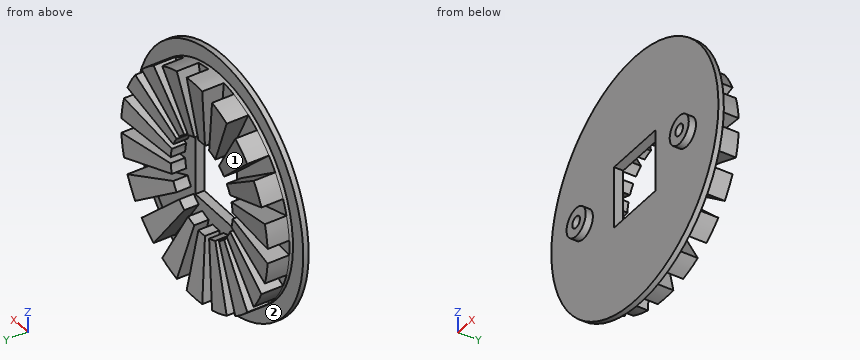
```python
from build123d import *

# Parameters (mm, degrees)
SKETCH2_R           = 15.35
BOSS_EXTRUDE3_DEPTH = 1.25
SKETCH5_W           = 8.7
SKETCH5_H           = 8.7
CUT_EXTRUDE3_DEPTH  = 1.25
BOSS_EXTRUDE4_DEPTH = 4.25
SKETCH1_R           = 17.5
SKETCH1_R_2         = 15.35
BOSS_EXTRUDE5_DEPTH = 0.75
SKETCH8_R           = 2
SKETCH8_R_2         = 0.8
BOSS_EXTRUDE6_DEPTH = 1


with BuildPart() as part:
    # Sketch2 → Boss-Extrude3 (new body)
    with BuildSketch(Plane(origin=(0, 0, 0), x_dir=(1, 0, 0), z_dir=(0, 1, 0))):
        with Locations(Location((0, 0, 0), (0, 0, 270))):
            Circle(SKETCH2_R)
    extrude(amount=BOSS_EXTRUDE3_DEPTH)

    # Sketch5 → Cut-Extrude3 (cut)
    with BuildSketch(Plane(origin=(0, 0, 0), x_dir=(-1, 0, 0), z_dir=(0, 1, 0))):
        Rectangle(SKETCH5_W, SKETCH5_H)
    extrude(amount=CUT_EXTRUDE3_DEPTH, mode=Mode.SUBTRACT)

    # Sketch3 → Boss-Extrude4 (add)
    with BuildSketch(Plane(origin=(0, 0, 0), x_dir=(1, 0, 0), z_dir=(0, 1, 0))):
        with BuildLine():
            Line((-1.631153495, 15.263087442), (-0.690716464, 6.463196637))
            ThreePointArc((-0.690716464, 6.463196637), (0, 6.5), (0.690716464, 6.463196637))
            Line((0.690716464, 6.463196637), (1.631153495, 15.263087442))
            ThreePointArc((1.631153495, 15.263087442), (0, 15.35), (-1.631153495, 15.263087442))
        make_face()
        with BuildLine():
            Line((3.687500452, 14.900497992), (1.561482276, 6.30965713))
            ThreePointArc((1.561482276, 6.30965713), (2.223130932, 6.108002035), (2.859604604, 5.837179242))
            Line((2.859604604, 5.837179242), (6.753066257, 13.784723288))
            ThreePointArc((6.753066257, 13.784723288), (5.2500092, 14.424281729), (3.687500452, 14.900497992))
        make_face()
        with BuildLine():
            Line((8.561387423, 12.740688576), (3.625343208, 5.395079853))
            ThreePointArc((3.625343208, 5.395079853), (4.178119463, 4.97928888), (4.683582226, 4.507111884))
            Line((4.683582226, 4.507111884), (11.060459564, 10.643718064))
            ThreePointArc((11.060459564, 10.643718064), (9.866789809, 11.758782202), (8.561387423, 12.740688576))
        make_face()
        with BuildLine():
            Line((12.402644718, 9.044164085), (5.251934245, 3.829776323))
            ThreePointArc((5.251934245, 3.829776323), (5.629165125, 3.25), (5.942650709, 2.633420314))
            Line((5.942650709, 2.633420314), (14.033798213, 6.218923357))
            ThreePointArc((14.033798213, 6.218923357), (13.293489948, 7.675), (12.402644718, 9.044164085))
        make_face()
        with BuildLine():
            Line((14.747960016, 4.256779928), (6.245064502, 1.802545246))
            ThreePointArc((6.245064502, 1.802545246), (6.401250395, 1.128713155), (6.484947812, 0.442099389))
            Line((6.484947812, 0.442099389), (15.31445368, 1.044034712))
            ThreePointArc((15.31445368, 1.044034712), (15.116799009, 2.665499527), (14.747960016, 4.256779928))
        make_face()
        with BuildLine():
            Line((15.31445368, -1.044034712), (6.484947812, -0.442099389))
            ThreePointArc((6.484947812, -0.442099389), (6.401250395, -1.128713155), (6.245064502, -1.802545246))
            Line((6.245064502, -1.802545246), (14.747960016, -4.256779928))
            ThreePointArc((14.747960016, -4.256779928), (15.116799009, -2.665499527), (15.31445368, -1.044034712))
        make_face()
        with BuildLine():
            Line((14.033798213, -6.218923357), (5.942650709, -2.633420314))
            ThreePointArc((5.942650709, -2.633420314), (5.629165125, -3.25), (5.251934245, -3.829776323))
            Line((5.251934245, -3.829776323), (12.402644718, -9.044164085))
            ThreePointArc((12.402644718, -9.044164085), (13.293489948, -7.675), (14.033798213, -6.218923357))
        make_face()
        with BuildLine():
            Line((11.060459564, -10.643718064), (4.683582226, -4.507111884))
            ThreePointArc((4.683582226, -4.507111884), (4.178119463, -4.97928888), (3.625343208, -5.395079853))
            Line((3.625343208, -5.395079853), (8.561387423, -12.740688576))
            ThreePointArc((8.561387423, -12.740688576), (9.866789809, -11.758782202), (11.060459564, -10.643718064))
        make_face()
        with BuildLine():
            Line((6.753066257, -13.784723288), (2.859604604, -5.837179242))
            ThreePointArc((2.859604604, -5.837179242), (2.223130932, -6.108002035), (1.561482276, -6.30965713))
            Line((1.561482276, -6.30965713), (3.687500452, -14.900497992))
            ThreePointArc((3.687500452, -14.900497992), (5.2500092, -14.424281729), (6.753066257, -13.784723288))
        make_face()
        with BuildLine():
            Line((1.631153495, -15.263087442), (0.690716464, -6.463196637))
            ThreePointArc((0.690716464, -6.463196637), (0, -6.5), (-0.690716464, -6.463196637))
            Line((-0.690716464, -6.463196637), (-1.631153495, -15.263087442))
            ThreePointArc((-1.631153495, -15.263087442), (0, -15.35), (1.631153495, -15.263087442))
        make_face()
        with BuildLine():
            Line((-3.687500452, -14.900497992), (-1.561482276, -6.30965713))
            ThreePointArc((-1.561482276, -6.30965713), (-2.223130932, -6.108002035), (-2.859604604, -5.837179242))
            Line((-2.859604604, -5.837179242), (-6.753066257, -13.784723288))
            ThreePointArc((-6.753066257, -13.784723288), (-5.2500092, -14.424281729), (-3.687500452, -14.900497992))
        make_face()
        with BuildLine():
            Line((-8.561387423, -12.740688576), (-3.625343208, -5.395079853))
            ThreePointArc((-3.625343208, -5.395079853), (-4.178119463, -4.97928888), (-4.683582226, -4.507111884))
            Line((-4.683582226, -4.507111884), (-11.060459564, -10.643718064))
            ThreePointArc((-11.060459564, -10.643718064), (-9.866789809, -11.758782202), (-8.561387423, -12.740688576))
        make_face()
        with BuildLine():
            Line((-12.402644718, -9.044164085), (-5.251934245, -3.829776323))
            ThreePointArc((-5.251934245, -3.829776323), (-5.629165125, -3.25), (-5.942650709, -2.633420314))
            Line((-5.942650709, -2.633420314), (-14.033798213, -6.218923357))
            ThreePointArc((-14.033798213, -6.218923357), (-13.293489948, -7.675), (-12.402644718, -9.044164085))
        make_face()
        with BuildLine():
            Line((-14.747960016, -4.256779928), (-6.245064502, -1.802545246))
            ThreePointArc((-6.245064502, -1.802545246), (-6.401250395, -1.128713155), (-6.484947812, -0.442099389))
            Line((-6.484947812, -0.442099389), (-15.31445368, -1.044034712))
            ThreePointArc((-15.31445368, -1.044034712), (-15.116799009, -2.665499527), (-14.747960016, -4.256779928))
        make_face()
        with BuildLine():
            Line((-15.31445368, 1.044034712), (-6.484947812, 0.442099389))
            ThreePointArc((-6.484947812, 0.442099389), (-6.401250395, 1.128713155), (-6.245064502, 1.802545246))
            Line((-6.245064502, 1.802545246), (-14.747960016, 4.256779928))
            ThreePointArc((-14.747960016, 4.256779928), (-15.116799009, 2.665499527), (-15.31445368, 1.044034712))
        make_face()
        with BuildLine():
            Line((-14.033798213, 6.218923357), (-5.942650709, 2.633420314))
            ThreePointArc((-5.942650709, 2.633420314), (-5.629165125, 3.25), (-5.251934245, 3.829776323))
            Line((-5.251934245, 3.829776323), (-12.402644718, 9.044164085))
            ThreePointArc((-12.402644718, 9.044164085), (-13.293489948, 7.675), (-14.033798213, 6.218923357))
        make_face()
        with BuildLine():
            Line((-11.060459564, 10.643718064), (-4.683582226, 4.507111884))
            ThreePointArc((-4.683582226, 4.507111884), (-4.178119463, 4.97928888), (-3.625343208, 5.395079853))
            Line((-3.625343208, 5.395079853), (-8.561387423, 12.740688576))
            ThreePointArc((-8.561387423, 12.740688576), (-9.866789809, 11.758782202), (-11.060459564, 10.643718064))
        make_face()
        with BuildLine():
            Line((-6.753066257, 13.784723288), (-2.859604604, 5.837179242))
            ThreePointArc((-2.859604604, 5.837179242), (-2.223130932, 6.108002035), (-1.561482276, 6.30965713))
            Line((-1.561482276, 6.30965713), (-3.687500452, 14.900497992))
            ThreePointArc((-3.687500452, 14.900497992), (-5.2500092, 14.424281729), (-6.753066257, 13.784723288))
        make_face()
    extrude(amount=BOSS_EXTRUDE4_DEPTH)

    # Sketch7 → Cut-Revolve1 (revolve, cut)
    with BuildSketch(Plane.XY, mode=Mode.PRIVATE) as cut_revolve1_sk:
        Polygon((6.5, 3.25), (15.31445368, 4.25), (6.5, 4.25), align=None)
    revolve(cut_revolve1_sk.sketch.rotate(Axis((0, 3.25, 0), (0, 1, 0)), 83.9), axis=Axis((0, 3.25, 0), (0, 1, 0)), mode=Mode.SUBTRACT)

    # Sketch1 → Boss-Extrude5 (add)
    with BuildSketch(Plane(origin=(0, 0, 0), x_dir=(1, 0, 0), z_dir=(0, 1, 0))):
        with Locations(Location((0, 0, 0), (0, 0, 270))):
            Circle(SKETCH1_R)
        with Locations(Location((0, 0, 0), (0, 0, 83.9))):
            Circle(SKETCH1_R_2, mode=Mode.SUBTRACT)
    extrude(amount=BOSS_EXTRUDE5_DEPTH)

    # Sketch8 → Boss-Extrude6 (add)
    # profile 1 of 2: a face of its own
    with BuildSketch(Plane(origin=(0, 0, 0), x_dir=(1, 0, 0), z_dir=(0, 1, 0))):
        with Locations(Location((-10.8, 0, 0), (0, 0, 270))):
            Circle(SKETCH8_R)
        with Locations(Location((-10.8, 0, 0), (0, 0, 270))):
            Circle(SKETCH8_R_2, mode=Mode.SUBTRACT)
    # profile 2 of 2: a face of its own
    with BuildSketch(Plane(origin=(0, 0, 0), x_dir=(1, 0, 0), z_dir=(0, 1, 0))):
        with Locations(Location((10.8, 0, 0), (0, 0, 90))):
            Circle(SKETCH8_R)
        with Locations(Location((10.8, 0, 0), (0, 0, 270))):
            Circle(SKETCH8_R_2, mode=Mode.SUBTRACT)
    extrude(amount=-BOSS_EXTRUDE6_DEPTH)


solid = part.part
```
Could you check a few things on this model? Use its own coordinates, in mm. Face numbers are marked on the shaded views. Round coordinates to 2 decimals unless told otherwise and drop trailing zeros. Loops run counter-clockwise (first coordinate to the right, second up) from the corner with the lowest first, then second, coordinate; pieces in that order, holes last. Notation, with made-up numbers: (-13.5, 50.25) - (42.5, 50.25) arc R26 ccw to (42.5, 83.25) - close; hole circle Ø1 at (-37, -20.5). An arc over 180 degrees is marked (long way). Answer in a Markdown table with one row per item. Add a question column.
(1) If we mould it in two halves opening along X, with no side actions, what happens to the marked faces 1 and 2? For each: pulls with the +X half, pulls with the -X half, needs draft (parallel to the pull), parting line crosses it, or undercut.
(2) If we section it at B-B (y = 2.35): State how many separate pieces and enclosed holes the cut face has, plus the area to 3 significant figures.
(3) I'm going to push flat-ended pins straight in: pin 1 (2 mm diameter, centred on y = 1, z = -11, fed in from -X); pin 2 (1.5 mm diameter, centred on x = -2.5, y = 0.5, fed in from +Z); pin 3 (4 mm diameter, centred on x = -5, z = -8.5, fed in from -Y); pin 4 (1.8 mm diameter, centred on x = 10.8, z = 0, fed in from -Y). Where does each tip first touch, or does it pass through?
(4) If we section it at A-A (z = 0): Please give me the cut outline in (x, y), plus the area to 3 significant figures.
(5) I need wall thicknesses on line 1 along X through (y, z) = (-0.4, 0); line 2 along Z through (x, y) = (12, 2.2); line 3 along Z through (x, y) = (-10.5, 3.2). Which ranges of each line are inside material? Lowest first, please.
Model answer:
| question | item | result |
|---|---|---|
| 1 | face 1 | undercut |
| 1 | face 2 | needs draft |
| 2 | separate pieces | 18 |
| 2 | enclosed holes | 0 |
| 2 | area | 371 mm² |
| 3 | pin 1 | stops at x = -14.34 |
| 3 | pin 2 | stops at z = 17.41 |
| 3 | pin 3 | stops at y = 0 |
| 3 | pin 4 | stops at y = -1 |
| 4 | outline | (-17.5, 0) - (-12.8, 0) - (-12.8, -1) - (-11.6, -1) - (-11.6, 0) - (-10, 0) - (-10, -1) - (-8.8, -1) - (-8.8, 0) - (-4.35, 0) - (-4.35, 1.25) - (-15.35, 1.25) - (-15.35, 0.75) - (-17.5, 0.75) - close; (4.35, 0) - (8.8, 0) - (8.8, -1) - (10, -1) - (10, 0) - (11.6, 0) - (11.6, -1) - (12.8, -1) - (12.8, 0) - (17.5, 0) - (17.5, 0.75) - (15.35, 0.75) - (15.35, 1.25) - (4.35, 1.25) - close |
| 4 | area | 35.5 mm² |
| 5 | line 1 | x = -12.8 to -11.6, -10 to -8.8, 8.8 to 10, 11.6 to 12.8 |
| 5 | line 2 | z = -8.75 to -5.32, -3.46 to -0.82, 0.82 to 3.46, 5.32 to 8.75 |
| 5 | line 3 | z = -11.2 to -10.1, -7.66 to -4.65, -3.03 to -0.72, 0.72 to 3.03, 4.65 to 7.66, 10.1 to 11.2 |
